Source: CAD feature listing. Evaluate the final solid. Frame: model axes, mm. Give positions to 0.01 mm unless a question says otherwise; leave off trailing zeros. Order: outer loops, then holes, each group sorted by start corner. A loop starts at its lowest first (then second) coordinate and runs counter-clockwise, first axis right, second up.
1) Material intervals for line 1 (Y direction, x = -10, z = 1.15); line 2 (Y direction, x = -30.5, z = 0.6); line 3 (X direction, y = 45, z = 0.7), sorted ascending.
2) Section A-A, the plane x = -14. Return loops of the section in (y, z).
3) Section D-D, the plane x = -23. Return loops of the section in (y, z).
4) Draft query along X for faces 1 (the face through (-52.88, 60.23, 0.8)), 2 (the face through (-29, 45, 0)). Return one class per face: released by +X, released by -X, zero draft, split by the parting line, or undercut.
5) Section B-B, the plane z = 0.75. Return loops of the section in (x, y) (3 decimals).
6) Section C-C, the plane y = 21. Return loops of the section in (x, z), plus the area to 3 significant figures.
7) First-contact query: P1, Ø6, axis at x = -41.5, y = 52.5, coming from the -Z side; P2, Ø0.5, axis at y = 87, z = 0.5, coming from the +X side; P3, Ø0.5, axis at x = -58, z = 1, coming from the -Y side; P4, Ø0.5, axis at y = 23, z = 0.5, coming from the -X side. Flat tips, straight axial feed; report the tip coordinate or a pass-through.
```python
from build123d import *

# Parameters (mm, degrees)
BOSS_EXTRUDE1_DEPTH = 1.5748
SKETCH2_R           = 1.397
BOSS_EXTRUDE2_DEPTH = 1.5748


with BuildPart() as part:
    # Sketch1 → Boss-Extrude1 (new body)
    with BuildSketch(Plane.XY):
        Polygon((3.048, 84.963), (0, 84.963), (0, 88.011), (-56.134, 88.011), (-56.134, 84.963), (-59.182, 84.963), (-59.182, 72.263), (-56.134, 72.263), (-56.134, 64.77), (0, 64.77), (0, 72.263), (3.048, 72.263), align=None)
    extrude(amount=BOSS_EXTRUDE1_DEPTH)

    # Sketch2 → Boss-Extrude2 (add)
    with BuildSketch(Plane.XY.offset(1.5748)):
        Polygon((-36.6014, 0), (-36.6014, 5.08), (-19.558, 5.08), (-19.558, 0), (0, 0), (0, 42.672), (-21.082, 42.672), (-21.082, 46.99), (0, 46.99), (0, 64.77), (-56.134, 64.77), (-56.134, 0), align=None)
        with Locations((-52.578, 3.556)):
            Circle(SKETCH2_R, mode=Mode.SUBTRACT)
        with Locations((-3.556, 3.556)):
            Circle(SKETCH2_R, mode=Mode.SUBTRACT)
        with Locations((-52.578, 61.595)):
            Circle(SKETCH2_R, mode=Mode.SUBTRACT)
        with Locations((-3.556, 61.595)):
            Circle(SKETCH2_R, mode=Mode.SUBTRACT)
    extrude(amount=-BOSS_EXTRUDE2_DEPTH)


solid = part.part
```
From the geometry:
1. line 1: y = 0 to 42.67, 46.99 to 88.01
1. line 2: y = 5.08 to 88.01
1. line 3: x = -56.13 to -21.08
2. outline: (0, 0) - (42.67, 0) - (42.67, 1.57) - (0, 1.57) - close; (46.99, 0) - (88.01, 0) - (88.01, 1.57) - (46.99, 1.57) - close
3. outline: (5.08, 0) - (88.01, 0) - (88.01, 1.57) - (5.08, 1.57) - close
4. face 1: undercut
4. face 2: zero draft
5. outline: (-59.182, 72.263) - (-56.134, 72.263) - (-56.134, 0) - (-36.601, 0) - (-36.601, 5.08) - (-19.558, 5.08) - (-19.558, 0) - (0, 0) - (0, 42.672) - (-21.082, 42.672) - (-21.082, 46.99) - (0, 46.99) - (0, 72.263) - (3.048, 72.263) - (3.048, 84.963) - (0, 84.963) - (0, 88.011) - (-56.134, 88.011) - (-56.134, 84.963) - (-59.182, 84.963) - close; hole circle Ø2.794 at (-52.578, 3.556); hole circle Ø2.794 at (-52.578, 61.595); hole circle Ø2.794 at (-3.556, 3.556); hole circle Ø2.794 at (-3.556, 61.595)
6. outline: (-56.13, 0) - (0, 0) - (0, 1.57) - (-56.13, 1.57) - close
6. area: 88.4 mm2
7. P1: stops at z = 0
7. P2: stops at x = 0
7. P3: stops at y = 72.26
7. P4: stops at x = -56.13
